Here's the drawing with two shaded views (mm, measured from the low corner). I have some questions. Coordinates: 2 decimals unless noted, no trailing zeros. Write each loop counter-clockwise with the first axis right and the second up, starting at its lowest first coordinate (ties: lowest second). Pieces come first, ordered by that corner, then holes. Notation, with made-up numbers: (88, 87) -> (120, 87) arc R32 ccw to (120, 126) -> close; hole circle Ø5 at (-19.5, -9). An arc over 180 degrees is marked (long way). Use a Markdown table: item, result. Add a question column.
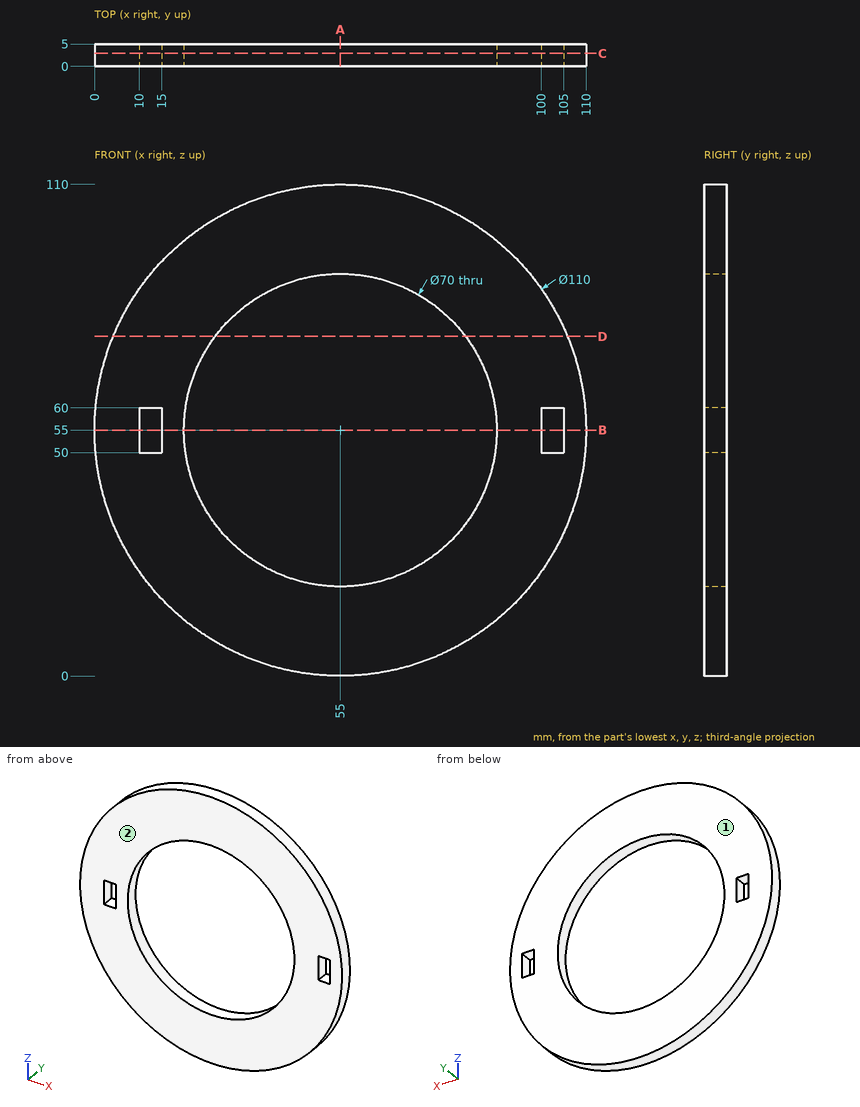
Q1. Will these pins go through, and if not, where does the flat tip stop? pin 1 (2.5 mm diameter, centred on y = 2.5, z = 56.5, fed in from -X); pin 2 (1.5 mm diameter, centred on x = 75, y = 4.5, fed in from +Z); pin 3 (1 mm diameter, centred on x = 48.5, y = 3, fed in from -Z); pin 4 (6 mm diameter, centred on x = 80.5, z = 71.5, fed in from +Y).
Q2. Suppose I cut it at A-A, the plane x = 55. Write out the boundary of the cut face in (y, z), and give its area (3 significant figures).
Q3. Suppose I cut it at C-C, the plane y = 2.9. Write out the boundary of the cut face in (x, z).
Q4. Thinking about a two-plate mould opening in Y: for the marked faces 1 and 2, which applies, released by +Y, released by -Y, zero draft, split by the parting line, or undercut?
Q5. Please list where these lines run through material, in increasing order: line 1 (X direction, y = 2.4, z = 55); line 2 (X direction, y = 3.8, z = 57); line 3 (Z direction, x = 78, y = 1.8).
Q6. Suppose I cut it at D-D, the plane z = 76. Write out the boundary of the cut face in (x, y), and give its area (3 significant figures).
Q7. Suppose I cut it at B-B, the plane z = 55. Write out the boundary of the cut face in (x, y), and give its area (3 significant figures).
Answer key:
| question | item | result |
|---|---|---|
| 1 | pin 1 | stops at x = 0 |
| 1 | pin 2 | stops at z = 106.52 |
| 1 | pin 3 | stops at z = 0.33 |
| 1 | pin 4 | passes through |
| 2 | outline | (0, 0) -> (5, 0) -> (5, 20) -> (0, 20) -> close; (0, 90) -> (5, 90) -> (5, 110) -> (0, 110) -> close |
| 2 | area | 200 mm^2 |
| 3 | outline | circle Ø110 at (55, 55); hole (10, 50) -> (15, 50) -> (15, 60) -> (10, 60) -> close; hole circle Ø70 at (55, 55); hole (100, 50) -> (105, 50) -> (105, 60) -> (100, 60) -> close |
| 4 | face 1 | released by +Y |
| 4 | face 2 | released by -Y |
| 5 | line 1 | x = 0 to 10, 15 to 20, 90 to 100, 105 to 110 |
| 5 | line 2 | x = 0.04 to 10, 15 to 20.06, 89.94 to 100, 105 to 109.96 |
| 5 | line 3 | z = 5.04 to 28.62, 81.38 to 104.96 |
| 6 | outline | (4.17, 0) -> (27, 0) -> (27, 5) -> (4.17, 5) -> close; (83, 0) -> (105.83, 0) -> (105.83, 5) -> (83, 5) -> close |
| 6 | area | 228 mm^2 |
| 7 | outline | (0, 0) -> (10, 0) -> (10, 5) -> (0, 5) -> close; (15, 0) -> (20, 0) -> (20, 5) -> (15, 5) -> close; (90, 0) -> (100, 0) -> (100, 5) -> (90, 5) -> close; (105, 0) -> (110, 0) -> (110, 5) -> (105, 5) -> close |
| 7 | area | 150 mm^2 |
